Model file for the job. Use its own axes, mm. A direction names the side the tool comes from. Coordinates: 2 decimals unless noted, no trailing zeros. Order: outer loops, then holes, each group sorted by start corner. A loop starts at its lowest first (then second) coordinate and runs counter-clockwise, first axis right, second up. Notation, with made-up numbers: M 47.5,-19.5 L 74.5,-19.5 A27 ccw 74.5,8.5 Z; hole C -17,-35.5 d5. An arc over 180 degrees is marked long. Return JSON: item names as keys, results as strings.
```python
from build123d import *

# Parameters (mm, degrees)
F0_W     = 151.971087
F0_H     = 90.071138
F1_DEPTH = 25.4
F2_R     = 24.678934
F3_DEPTH = 38.1
F5_DEPTH = 90.072138


with BuildPart() as f1:
    # F0 (on Top) → F1 (new body)
    with BuildSketch(Plane.XY):
        with Locations((-0.095821, -3.162073)):
            Rectangle(F0_W, F0_H)
    extrude(amount=F1_DEPTH)

    # F2 (on face) → F3 (join)
    with BuildSketch(Plane.XY.offset(25.4)):
        with Locations((0, -0.479101)):
            Circle(F2_R)
    extrude(amount=F3_DEPTH)

    # F4 (on face) → F5 (cut, through all)
    with BuildSketch(Plane.XZ.offset(48.197642)):
        Polygon((29.129392, 74.644059), (-56.150731, 66.211872), (38.519785, 38.423963), align=None)
    extrude(amount=-F5_DEPTH, mode=Mode.SUBTRACT)


solid = f1.part
```
Item 1: Saw through at D-D (x = 28). Write the cut outline in (y, z).
Check result:
{"outline": "M -48.2,0 L 41.87,0 L 41.87,25.4 L -48.2,25.4 Z"}
Item 2: Saw through at C-C (z = 45.5). Write the cut outline in (x, y), and give its area (3 significant figures).
Check result:
{"outline": "M 14.41,-20.51 L 14.41,19.55 A24.68 ccw long Z", "area": "1,630 mm2"}
Item 3: Saw through at A-A (y = 9.5). Write the cut outline in (x, z), and give its area (3 significant figures).
Check result:
{"outline": "M -76.08,0 L 75.89,0 L 75.89,25.4 L 22.57,25.4 L 22.57,43.11 L -22.57,56.36 L -22.57,25.4 L -76.08,25.4 Z", "area": "4,960 mm2"}
Item 4: Drop flat-ended pins along their axis: pin 1 Ø3 at (y, z) = (-11, 46.5) entering from -X; pin 2 Ø3 at (x, y) = (-32.5, 14.5) entering from +Z; pin 3 Ø1 at (y, z) = (-13, 42) entering from -X. Give the stop position or say it passes through.
Check result:
{"pin 1": "stops at x = -22.97", "pin 2": "stops at z = 25.4", "pin 3": "stops at x = -21.55"}
Item 5: 3-axis set-ups, long thin cutter, end or side, ignore diameter. For faces 1 (the cylindrical face through (-24.655, 0.606, 37.572)), 2 (the flat face through (-76.081, -4, 13)): which of +Z, -Z, +X, -X, +Y, -Y reach the whole face in a straight line?
Check result:
{"face 1": "+Z", "face 2": "+Z, -Z, -X, +Y, -Y"}
Item 6: Saw through at B-B (x = 0). Write the cut outline in (y, z).
Check result:
{"outline": "M -48.2,0 L 41.87,0 L 41.87,25.4 L 24.2,25.4 L 24.2,49.73 L -25.16,49.73 L -25.16,25.4 L -48.2,25.4 Z"}
Item 7: Wall check: line 1 (Z direction, x = 50, y = 35.5); line 2 (Y direction, x = -21.5, z = 30.5); line 3 (Y direction, x = -9, z = 51). Give the ranges that are in metal, low to high.
Check result:
{"line 1": "z = 0 to 25.4", "line 2": "y = -12.6 to 11.64", "line 3": "y = -23.46 to 22.5"}
